```python
from build123d import *

# Parameters (mm, degrees)
SKETCH1_R           = 5
BOSS_EXTRUDE1_DEPTH = 5


with BuildPart() as part:
    # Sketch1 → Boss-Extrude1 (new body)
    with BuildSketch(Plane(origin=(0, 0, 0), x_dir=(1, 0, 0), z_dir=(0, 1, 0))):
        with BuildLine():
            Line((-10, 0), (-10, 100))
            ThreePointArc((-10, 100), (0, 110), (10, 100))
            Line((10, 100), (10, 0))
            ThreePointArc((10, 0), (0, -10), (-10, 0))
        make_face()
        Circle(SKETCH1_R, mode=Mode.SUBTRACT)
        with Locations((0, 100)):
            Circle(SKETCH1_R, mode=Mode.SUBTRACT)
        with BuildLine():
            Line((5, 85), (5, 15))
            ThreePointArc((5, 15), (0, 10), (-5, 15))
            Line((-5, 15), (-5, 85))
            ThreePointArc((-5, 85), (0, 90), (5, 85))
        make_face(mode=Mode.SUBTRACT)
    extrude(amount=BOSS_EXTRUDE1_DEPTH)


solid = part.part
```
For this review, take the finished solid that the model builds, in its own axes (mm). A direction names the side the tool comes from. Give positions to 0.01 mm unless a question says otherwise; leave off trailing zeros. Order: outer loops, then holes, each group sorted by start corner. A loop starts at its lowest first (then second) coordinate and runs counter-clockwise, first axis right, second up.
1) Insertion check: pin 1 (2 mm diameter, centred on x = 5.5, y = 2.5, fed in from -Z); pin 2 (1.5 mm diameter, centred on x = 4, y = 1.5, fed in from -Z); pin 3 (1.5 mm diameter, centred on x = -5, y = 3.5, fed in from +Z). Each pin has a flat end and moves straight along its axis. Give the tip position at first contact, or say it passes through.
2) Take a section at A-A (z = -3). Give the boundary of the cut face in (x, y).
3) The part is to be moulded in two halves that separate along Z. For faces 1 (the face through (-10, 2, -49)), 2 (the face through (0, 2, -110)), 3 (the face through (5, 2, -50)), say which applies: released by +Z, released by -Z, zero draft, split by the parting line, or undercut.
4) Take a section at D-D (z = -49). Give the boundary of the cut face in (x, y), then the cut area to 3 significant figures.
5) Wall thickness on line 1 (Z direction, x = 0, y = 2.15); line 2 (X direction, y = 2.35, z = -100); line 3 (Z direction, x = -2, y = 4.1): over which ranges is each line inside the solid? List them lowest first.
6) For faces 4 (the face through (0, 2, 10)), 5 (the face through (0, 2, -10)), list the 3-axis set-ups (+Z, -Z, +X, -X, +Y, -Y) from which the entire face can be reached by the end or side of a thin tool; tool diameter is ignored.
7) Take a section at C-C (x = 4). Give the boundary of the cut face in (y, z).
8) Take a section at B-B (y = 0.9). Give the boundary of the cut face in (x, z).
Derived:
1. pin 1: stops at z = -108.93
1. pin 2: stops at z = -109.46
1. pin 3: stops at z = 9.05
2. outline: (-10, 0) - (-4, 0) - (-4, 5) - (-10, 5) - close; (4, 0) - (10, 0) - (10, 5) - (4, 5) - close
3. face 1: zero draft
3. face 2: released by -Z
3. face 3: undercut
4. outline: (-10, 0) - (-5, 0) - (-5, 5) - (-10, 5) - close; (5, 0) - (10, 0) - (10, 5) - (5, 5) - close
4. area: 50.0 mm2
5. line 1: z = -110 to -105, -95 to -90, -10 to -5, 5 to 10
5. line 2: x = -10 to -5, 5 to 10
5. line 3: z = -109.8 to -104.58, -95.42 to -89.58, -10.42 to -4.58, 4.58 to 9.8
6. face 4: +Z, +Y, -Y
6. face 5: +Y, -Y
7. outline: (0, -109.17) - (5, -109.17) - (5, -103) - (0, -103) - close; (0, -97) - (5, -97) - (5, -88) - (0, -88) - close; (0, -12) - (5, -12) - (5, -3) - (0, -3) - close; (0, 3) - (5, 3) - (5, 9.17) - (0, 9.17) - close
8. outline: (-10, -100) arc R10 ccw to (10, -100) - (10, 0) arc R10 ccw to (-10, 0) - close; hole circle Ø10 at (0, -100); hole (-5, -85) arc R5 ccw to (5, -85) - (5, -15) arc R5 ccw to (-5, -15) - close; hole circle Ø10 at (0, 0)
